```python
from build123d import *

# Parameters (mm, degrees)
F1_DEPTH = 20
F2_R     = 10
F3_DEPTH = 20


with BuildPart() as f1:
    # F0 (on Front) → F1 (new body)
    with BuildSketch(Plane.XZ):
        with BuildLine():
            ThreePointArc((24.206146, -6.25), (24.800742, -3.150107), (25, 0))
            ThreePointArc((25, 0), (24.800742, 3.150107), (24.206146, 6.25))
            ThreePointArc((24.206146, 6.25), (0, 25), (-24.206146, 6.25))
            ThreePointArc((-24.206146, 6.25), (-25, 0), (-24.206146, -6.25))
            ThreePointArc((-24.206146, -6.25), (0, -25), (24.206146, -6.25))
        make_face()
        with BuildLine():
            ThreePointArc((-24.206146, 6.25), (0, 25), (24.206146, 6.25))
            Line((24.206146, 6.25), (9.682458, 62.5))
            ThreePointArc((9.682458, 62.5), (9.920297, 61.260043), (10, 60))
            ThreePointArc((10, 60), (-1.260043, 50.079703), (-9.682458, 62.5))
            Line((-9.682458, 62.5), (-24.206146, 6.25))
        make_face()
        with BuildLine():
            Line((9.682458, -62.5), (24.206146, -6.25))
            ThreePointArc((24.206146, -6.25), (0, -25), (-24.206146, -6.25))
            Line((-24.206146, -6.25), (-9.682458, -62.5))
            ThreePointArc((-9.682458, -62.5), (-1.260043, -50.079703), (10, -60))
            ThreePointArc((10, -60), (9.920297, -61.260043), (9.682458, -62.5))
        make_face()
        with BuildLine():
            ThreePointArc((10, 60), (9.920297, 61.260043), (9.682458, 62.5))
            ThreePointArc((9.682458, 62.5), (0, 70), (-9.682458, 62.5))
            ThreePointArc((-9.682458, 62.5), (-1.260043, 50.079703), (10, 60))
        make_face()
        with BuildLine():
            ThreePointArc((-9.682458, -62.5), (0, -70), (9.682458, -62.5))
            ThreePointArc((9.682458, -62.5), (9.920297, -61.260043), (10, -60))
            ThreePointArc((10, -60), (-1.260043, -50.079703), (-9.682458, -62.5))
        make_face()
    extrude(amount=F1_DEPTH)

    # F2 (on face) → F3 (join)
    with BuildSketch(Plane(origin=(0, 0, 0), x_dir=(-1, 0, 0), z_dir=(0, 1, 0))):
        Circle(F2_R)
    extrude(amount=F3_DEPTH)


solid = f1.part
```
Check sheet for the modelled part. Datum: model origin and axes. Units: mm. A direction names the side the tool comes from. Give positions to 0.01 mm unless a question says otherwise; leave off trailing zeros. Order: outer loops, then holes, each group sorted by start corner. A loop starts at its lowest first (then second) coordinate and runs counter-clockwise, first axis right, second up. Notation, with made-up numbers: M -26,8.25 L 13,8.25 A32 cw 13,40.25 Z; hole C 73.5,12.5 d9. An arc over 180 degrees is marked long. Answer in a Markdown table with one row per item.
1) Thickness scan on L1, parallel to Y at x = -6, z = -45; L2, parallel to Z at x = 8.5, y = 7; L3, parallel to Z at x = 0, y = 3.5. Record the ranges inside material, lowest first. Write a range as [from, to].
Filled sheet:
| item | result |
|---|---|
| L1 | y = [-20, 0] |
| L2 | z = [-5.27, 5.27] |
| L3 | z = [-10, 10] |
2) Access from +Z, -Z, +X, -X, +Y, -Y to the whole of each face (thin tool, end or side, straight path). Record for faces 1 (the cylindrical face through (2.17, 9.86, -9.76)), 2 (the flat face through (17.046, -9.86, 33.981)).
Filled sheet:
| item | result |
|---|---|
| face 1 | +Y |
| face 2 | +Z, +X, +Y, -Y |
3) Cross-section at D-D, the plane x = -5.5. Enter the section's corners in (y, z), plus the area to 3 significant figures.
Filled sheet:
| item | result |
|---|---|
| outline | M -20,-68.35 L 0,-68.35 L 0,-8.35 L 20,-8.35 L 20,8.35 L 0,8.35 L 0,68.35 L -20,68.35 Z |
| area | 3,070 mm2 |
4) Cross-section at C-C, the plane z = -26.5. Enter the section's corners in (x, y).
Filled sheet:
| item | result |
|---|---|
| outline | M -18.98,-20 L 18.98,-20 L 18.98,0 L -18.98,0 Z |
5) Cross-section at B-B, the plane x = 0. Enter the section's corners in (y, z).
Filled sheet:
| item | result |
|---|---|
| outline | M -20,-70 L 0,-70 L 0,-10 L 20,-10 L 20,10 L 0,10 L 0,70 L -20,70 Z |
6) Gauge pin test, flat end, axial feed: P1, Ø15, axis at x = -12, z = -32, coming from the +Y side. Record the tip position at first contact, or that the pin passes through.
Filled sheet:
| item | result |
|---|---|
| P1 | stops at y = 0 |
7) Cross-section at A-A, the plane y = -3. Enter the section's corners in (x, z).
Filled sheet:
| item | result |
|---|---|
| outline | M -24.21,-6.25 L -9.68,-62.5 A10 ccw 9.68,-62.5 L 24.21,-6.25 A25 ccw 25,0 A25 ccw 24.21,6.25 L 9.68,62.5 A10 ccw -9.68,62.5 L -24.21,6.25 A25 ccw Z |
